Verification items for this drawing (mm, ordinates from the low corner). A direction names the side the tool comes from. Coordinates: 2 decimals unless noted, no trailing zeros. Write each loop counter-clockwise with the first axis right and the second up, starting at its lowest first coordinate (ties: lowest second). Pieces come first, ordered by that corner, then holes. Notation, with made-up numbers: M 28,12 L 66,12 A25 cw 66,26 Z; hole C -0.5,-25 d8. An arc over 180 degrees is marked long. Answer as CSV lines item,"result". Start each with the question number.
1) Draft check along Z on the marked faces 3, 4 and 5. Enter one of: +Z half, -Z half, draft (parallel to the pull), parting line (faces both ways), or undercut.
2) Section check B-B (z = 26.5). Record the cut outline in (x, y), and give its area (3 significant figures).
3) Material ranges on L1, parallel to X at y = 2.45, z = 5; L2, parallel to Z at x = 34, y = 2.45, recorded low to high. Write a range as [from, to].
4) Go/stop test with a flat-tipped pin: pin 1 Ø5 at (x, z) = (25, 35) entering from +Y. Record where the tip stops, or that it passes through.
5) Access from +Z, -Z, +X, -X, +Y, -Y to the whole of each face (thin tool, end or side, straight path). Record for the marked faces 1 and 2.
6) Section check A-A (x = 5). Record the cut outline in (y, z).
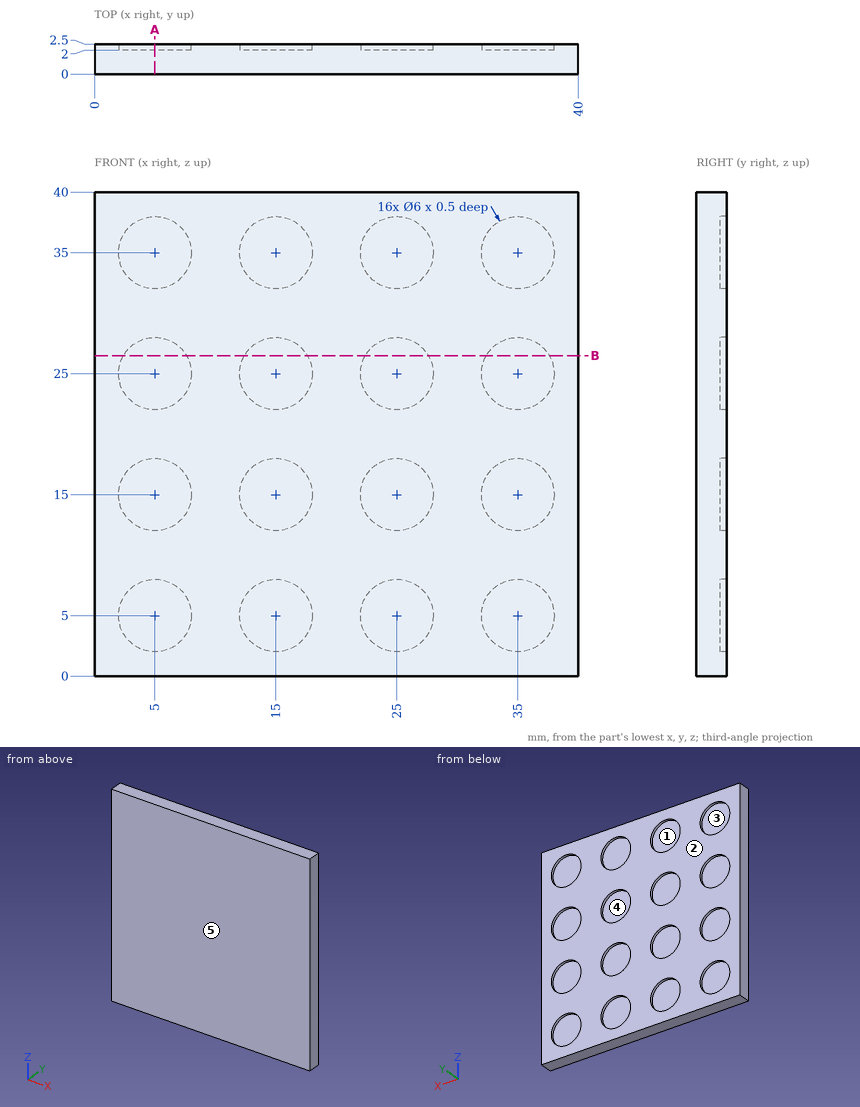
Results found:
1,face 3,"undercut"
1,face 4,"undercut"
1,face 5,"draft"
2,outline,"M 0,0 L 40,0 L 40,2.5 L 37.6,2.5 L 37.6,2 L 32.4,2 L 32.4,2.5 L 27.6,2.5 L 27.6,2 L 22.4,2 L 22.4,2.5 L 17.6,2.5 L 17.6,2 L 12.4,2 L 12.4,2.5 L 7.6,2.5 L 7.6,2 L 2.4,2 L 2.4,2.5 L 0,2.5 Z"
2,area,"89.6 mm2"
3,L1,"x = [0, 2], [8, 12], [18, 22], [28, 32], [38, 40]"
3,L2,"z = [0, 2.17], [7.83, 12.17], [17.83, 22.17], [27.83, 32.17], [37.83, 40]"
4,pin 1,"stops at y = 2"
5,face 1,"+Y"
5,face 2,"+Z, -Z, +X, -X, +Y"
6,outline,"M 0,0 L 2.5,0 L 2.5,2 L 2,2 L 2,8 L 2.5,8 L 2.5,12 L 2,12 L 2,18 L 2.5,18 L 2.5,22 L 2,22 L 2,28 L 2.5,28 L 2.5,32 L 2,32 L 2,38 L 2.5,38 L 2.5,40 L 0,40 Z"
